For this review, use the dimensioned drawing (mm, ordinates from the lowest corner) and the shaded views. A direction names the side the tool comes from. Coordinates: 2 decimals unless noted, no trailing zeros. Order: outer loops, then holes, each group sorted by start corner. A loop starts at its lowest first (then second) coordinate and runs counter-clockwise, first axis right, second up. Notation, with made-up numbers: M 37.25,31.5 L 93.25,31.5 A22 cw 93.25,69.5 Z; hole C 69.5,-22.5 d3. An arc over 180 degrees is marked long. Use CSV: the item, a comma, the result in double quotes.
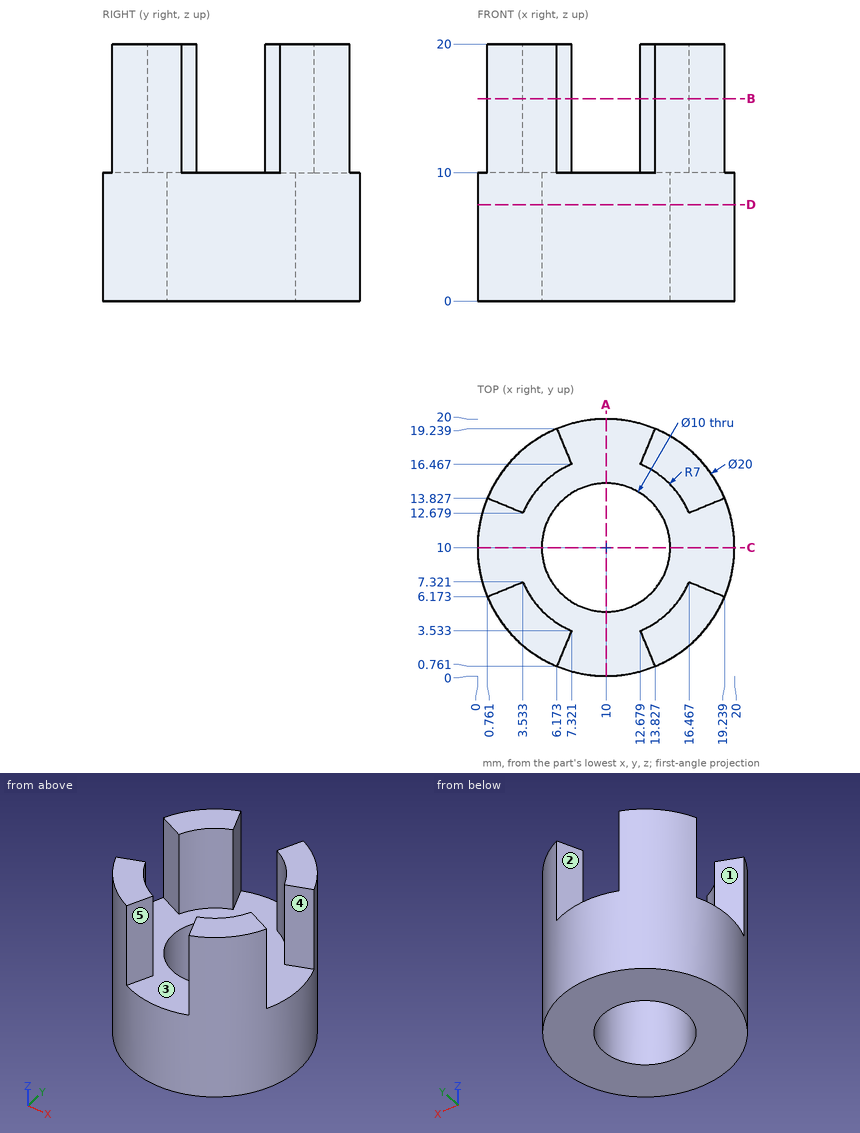
Item 1: For the marked faces 1, 2, 3, 4 and 5, list the 3-axis set-ups (+Z, -Z, +X, -X, +Y, -Y) from which the entire face can be reached by the end or side of a thin tool; tool diameter is ignored.
Solutions:
face 1,"+Z, -X"
face 2,"+Z, +Y"
face 3,"+Z"
face 4,"+Z, +X"
face 5,"+Z, -Y"
Item 2: To check wall thickness, follow line 1 along Y through (x, z) = (10, 2); line 2 along X through (y, z) = (17, 16); line 3 along Z through (x, y) = (17.5, 11.5). State the ranges of each line that lie inside material, in increasing order. Write a range as [from, to].
Solutions:
line 1,"[0, 5], [15, 20]"
line 2,"[2.86, 7.1], [12.9, 17.14]"
line 3,"[0, 10]"
Item 3: Clearance check with flat-ended pins moving along their axes: pin 1 Ø2 at (x, z) = (3.5, 2.5) entering from -Y; pin 2 Ø10 at (y, z) = (16.5, 12.5) entering from +X; pin 3 Ø4 at (x, z) = (3.5, 13) entering from +Y; pin 4 Ø3 at (x, z) = (8.5, 4) entering from +Y. State where each tip first meets the part, or that it passes through.
Solutions:
pin 1,"y = 1.65"
pin 2,"x = 19.76"
pin 3,"y = 18.93"
pin 4,"y = 20"
Item 4: Add section A-A on x = 10. State the section outline as (y, z) points.
Solutions:
outline,"M 0,0 L 5,0 L 5,10 L 0,10 Z; M 15,0 L 20,0 L 20,10 L 15,10 Z"
Item 5: Add section B-B on z = 15.75. State the section outline as (x, y) points, and give its area (3 significant figures).
Solutions:
outline,"M 0.76,6.17 A10 ccw 6.17,0.76 L 7.32,3.53 A7 cw 3.53,7.32 Z; M 0.76,13.83 L 3.53,12.68 A7 cw 7.32,16.47 L 6.17,19.24 A10 ccw Z; M 12.68,3.53 L 13.83,0.76 A10 ccw 19.24,6.17 L 16.47,7.32 A7 cw Z; M 12.68,16.47 A7 cw 16.47,12.68 L 19.24,13.83 A10 ccw 13.83,19.24 Z"
area,"80.1 mm^2"
Item 6: Add section D-D on z = 7.5. State the section outline as (x, y) points, and give its area (3 significant figures).
Solutions:
outline,"C 10,10 d20; hole C 10,10 d10"
area,"236 mm^2"
